Here's how the part is built. I have some questions about the finished solid (model axes, mm). A direction names the side the tool comes from. Round coordinates to 2 decimals unless told otherwise and drop trailing zeros. Loops run counter-clockwise (first coordinate to the right, second up) from the corner with the lowest first, then second, coordinate; pieces in that order, holes last. Notation, with made-up numbers: (-29, -33) -> (-24, -33) arc R21 ccw to (-24, -29) -> close; hole circle Ø8 at (38, -31.75). An arc over 180 degrees is marked (long way). Use one line per item in the form item = value. Start each with the question number.
Item 1: Thinking about a two-plate mould opening in X: for faces 4 (the face through (0, 1, 25)), 5 (the face through (-52, 54, 25)), 6 (the face through (-43.095, 1.521, 9.959)), 7 (the face through (-26, 2, 37.91)), which applies, released by +X, released by -X, zero draft, split by the parting line, or undercut?
Item 2: If I drill on L1, parallel to X at y = 21.5, z = 23.5; L2, parallel to Y at x = -8.5, z = 22; L3, parallel to Z at x = -9.5, y = 2, over which ranges is the centre line in solid material (lowest first)? Write a range as [from, to].
Item 3: If we section it at C-C (z = 39): Write out the boundary of the cut face in (x, y).
Item 4: If we section it at B-B (z = 25.5): Write out the boundary of the cut face in (x, y).
Item 5: If we section it at A-A (x = -14): Write out the boundary of the cut face in (y, z), then the cut area to 3 significant figures.
Item 6: For faces 1 (the face through (-50, 28, 25)), 2 (the face through (-8.903, 1.521, 40.051)), 3 (the face through (-26, 0, 25)), which set-ups out of +Z, -Z, +X, -X, +Y, -Y let a thin tool reach every point of the face, with its end or its side?
Item 7: I'm going to push flat-ended pins straight in: pin 1 Ø15 at (x, z) = (-37, 22) entering from +Y; pin 2 Ø8 at (y, z) = (12.5, 44) entering from +X; pin 3 Ø3 at (x, z) = (-16, 10) entering from -Y. Where does each tip first touch, or does it pass through?
Item 8: If we section it at D-D (x = -4): Write out the boundary of the cut face in (y, z).
Autodesk Inventor part; units mm, degrees
ref_plane "YZ Plane" through (0, 0, 0) normal (1, 0, 0) x (0, 1, 0)
ref_plane "XZ Plane" through (0, 0, 0) normal (0, 1, 0) x (-1, 0, 0)
ref_plane "XY Plane" through (0, 0, 0) normal (0, 0, 1) x (1, 0, 0)
sketch "Sketch1" plane through (0, 0, 0) normal (0, 1, 0) x (-1, 0, 0)
  line L0 (0, 0) -> (52.9999, 0)
  line L1 (52.9999, 0) -> (52.9999, 49.9999)
  line L2 (52.9999, 49.9999) -> (0, 49.9999)
  line L3 (0, 49.9999) -> (0, 0)
  dimension "d0" = 52.9999
  dimension "d1" = 49.9999
extrude "Extrusion1" add sketch "Sketch1" along normal blind 3
sketch "Sketch2" plane through (0, 3, 0) normal (0, 1, 0) x (1, 0, 0)
  line L0 (-52.9999, 0) -> (-52.9999, -49.9999)
  line L1 (0, 0) -> (-52.9999, 0)
  line L2 (-52.9999, -49.9999) -> (-49.9999, -49.9999)
  line L3 (-49.9999, -49.9999) -> (-49.9999, 0)
  line L4 (-49.9999, 0) -> (-52.9999, 0)
  line L5 (-52.9999, 0) -> (-52.9999, -49.9999)
  dimension "d4" = 3
extrude "Extrusion2" add sketch "Sketch2" along normal blind 50.9999
sketch "Sketch3" plane through (0, 3, 0) normal (0, 1, 0) x (1, 0, 0)
  line L0 (0, -49.9999) -> (0, 0)
  line L1 (0, -10.0051) -> (-11, -10.0051)
  circle A0 centre (-11, -10.0051) radius 2.1
  line L2 (-11, -10.0051) -> (-40.9999, -10.0051)
  circle A1 centre (-40.9999, -10.0051) radius 2.0955
  line L3 (-41.0003, -12.1006) -> (-11.0003, -12.1051)
  line L4 (-11.0003, -7.9051) -> (-41.0003, -7.9096)
  line L5 (0, -40.005) -> (-10.9982, -40.005)
  circle A2 centre (-10.9982, -40.005) radius 2.0955
  circle A3 centre (-41.0003, -40.005) radius 2.0955
  line L6 (-41.0003, -42.1005) -> (-10.9982, -42.1005)
  line L7 (-10.9982, -37.9095) -> (-41.0003, -37.9095)
  line L8 (-49.9999, -49.9999) -> (0, -49.9999)
  line L9 (0, 0) -> (-49.9999, 0)
  dimension "d7" = 11
  dimension "d8" = 4.2
  dimension "d9" = 29.9999
  dimension "d10" = 4.191
  dimension "d11" = 10.9982
  dimension "d12" = 4.191
  dimension "d13" = 4.191
  dimension "d14" = 29.9999
  dimension "d15" = 9.9949
  dimension "d16" = 10.0051
extrude "Extrusion3" cut sketch "Sketch3" against normal blind 12.5001
properties part number "Nema 3 Mounting"
Values found:
q1.face_4 = released by +X
q1.face_5 = zero draft
q1.face_6 = undercut
q1.face_7 = undercut
q2.L1 = [-53, -50]
q2.L2 = [0, 3]
q2.L3 = [0, 8.54], [11.47, 38.54], [41.47, 50]
q3.outline = (-53, 0) -> (-42.84, 0) -> (-42.84, 3) -> (-50, 3) -> (-50, 54) -> (-53, 54) -> close; (-9.16, 0) -> (0, 0) -> (0, 3) -> (-9.16, 3) -> close
q4.outline = (-53, 0) -> (0, 0) -> (0, 3) -> (-50, 3) -> (-50, 54) -> (-53, 54) -> close
q5.outline = (0, 0) -> (3, 0) -> (3, 7.91) -> (0, 7.91) -> close; (0, 12.1) -> (3, 12.1) -> (3, 37.91) -> (0, 37.91) -> close; (0, 42.1) -> (3, 42.1) -> (3, 50) -> (0, 50) -> close
q5.area = 125 mm2
q6.face_1 = +Z, -Z, +X, +Y
q6.face_2 = +Y, -Y
q6.face_3 = +Z, -Z, +X, -X, -Y
q7.pin_1 = 3
q7.pin_2 = -50
q7.pin_3 = through
q8.outline = (0, 0) -> (3, 0) -> (3, 50) -> (0, 50) -> close
